from build123d import *

# Parameters (mm, degrees)
SKETCH1_R           = 50
BOSS_EXTRUDE1_DEPTH = 80
BOSS_EXTRUDE2_START = 4
SKETCH1_3_R         = 56
SKETCH1_3_R_2       = 50
BOSS_EXTRUDE2_DEPTH = 4
SKETCH5_W           = 51
SKETCH5_H           = 28
BOSS_EXTRUDE4_DEPTH = 38
SKETCH6_W           = 47
SKETCH6_H           = 28
CUT_EXTRUDE2_DEPTH  = 36
SKETCH8_R           = 7.5
CUT_EXTRUDE3_DEPTH  = 51


with BuildPart() as part:
    # Sketch1 → Boss-Extrude1 (new body)
    with BuildSketch(Plane(origin=(0, 0, 0), x_dir=(1, 0, 0), z_dir=(0, 1, 0))):
        with Locations(Location((0, 0, 0), (0, 0, 270))):
            Circle(SKETCH1_R)
    extrude(amount=-BOSS_EXTRUDE1_DEPTH)

    # Sketch1_3 → Boss-Extrude2 (add)
    # profile 1 of 2: a face of its own
    with BuildSketch(Plane(origin=(0, 0, 0), x_dir=(1, 0, 0), z_dir=(0, 1, 0)).offset(BOSS_EXTRUDE2_START)):
        with Locations(Location((0, 0, 0), (0, 0, 270))):
            Circle(SKETCH1_3_R)
        with Locations(Location((0, 0, 0), (0, 0, 270))):
            Circle(SKETCH1_3_R_2, mode=Mode.SUBTRACT)
    # profile 2 of 2: a face of its own
    with BuildSketch(Plane(origin=(0, 0, 0), x_dir=(1, 0, 0), z_dir=(0, 1, 0)).offset(BOSS_EXTRUDE2_START)):
        with Locations(Location((0, 0, 0), (0, 0, 270))):
            Circle(SKETCH1_3_R_2)
    extrude(amount=-BOSS_EXTRUDE2_DEPTH)

    # Sketch5 → Boss-Extrude4 (add)
    with BuildSketch(Plane(origin=(0, 4, 0), x_dir=(1, 0, 0), z_dir=(0, 1, 0))):
        Rectangle(SKETCH5_W, SKETCH5_H)
    extrude(amount=BOSS_EXTRUDE4_DEPTH)

    # Sketch6 → Cut-Extrude2 (cut)
    with BuildSketch(Plane(origin=(0, 42, 0), x_dir=(1, 0, 0), z_dir=(0, 1, 0))):
        Rectangle(SKETCH6_W, SKETCH6_H)
    extrude(amount=-CUT_EXTRUDE2_DEPTH, mode=Mode.SUBTRACT)

    # Sketch8 → Cut-Extrude3 (cut)
    with BuildSketch(Plane(origin=(25.5, 0, 0), x_dir=(0, 0, -1), z_dir=(1, 0, 0))):
        with Locations((0, 42)):
            Circle(SKETCH8_R)
    extrude(amount=-CUT_EXTRUDE3_DEPTH, mode=Mode.SUBTRACT)


solid = part.part
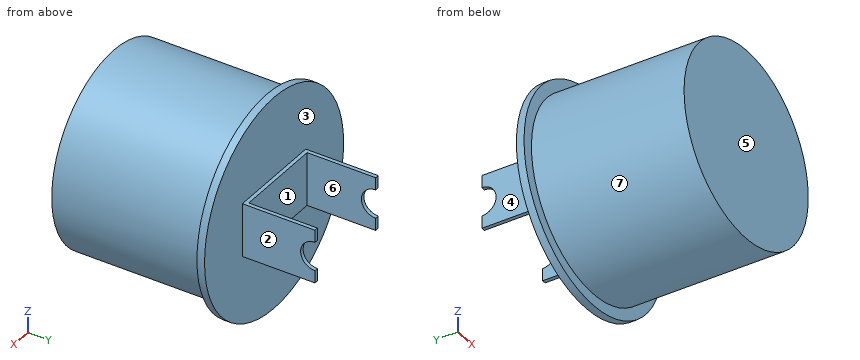
Part model, mm, in its own coordinate system. Face numbers are marked on the shaded views. A direction names the side the tool comes from. Give positions to 0.01 mm unless a question says otherwise; leave off trailing zeros. Order: outer loops, then holes, each group sorted by start corner. A loop starts at its lowest first (then second) coordinate and runs counter-clockwise, first axis right, second up. Notation, with made-up numbers: (-31.75, 36) - (4.25, 36) arc R28 cw to (4.25, 71) - close; hole circle Ø6 at (-25.5, 19.25). An arc over 180 degrees is marked (long way). One line per question, with ' | ' between items.
1. Band-saw the part on C-C on y = -57. List the corners of the cut face in (x, z).
Filled in:
outline: circle Ø100 at (0, 0)
2. Band-saw the part on D-D on z = 34. List the corners of the cut face in (x, y).
Filled in:
outline: (-44.5, 0) - (-36.66, 0) - (-36.66, -80) - (36.66, -80) - (36.66, 0) - (44.5, 0) - (44.5, 4) - (-44.5, 4) - close
3. Pull direction X, two halves, no side cores. Call the marked faces 1, 2 and 3: +X half, -X half, draft (parallel to the pull), parting line (faces both ways), or undercut.
Filled in:
face 1: undercut | face 2: +X half | face 3: draft
4. Drop flat-ended pins along their axis: P1, Ø8.5, axis at y = 28.5, z = 1, coming from the -X side; P2, Ø14, axis at x = 7.5, z = 0, coming from the +Y side; P3, Ø10, axis at y = -62.5, z = -30.5, coming from the -X side. Give the stop position or say it passes through.
Filled in:
P1: x = -25.5 | P2: y = 6 | P3: x = -43.01
5. Band-saw the part on A-A on x = 0. List the corners of the cut face in (y, z), then the cut area to 3 significant figures.
Filled in:
outline: (-80, -50) - (0, -50) - (0, -56) - (4, -56) - (4, -14) - (6, -14) - (6, 14) - (4, 14) - (4, 56) - (0, 56) - (0, 50) - (-80, 50) - close | area: 8,500 mm²
6. Drill centre lines: probe 1 along Y at (x, z) = (45.5, 30.5); probe 2 along Y at (x, z) = (7, -4); probe 3 along X at (y, z) = (-72.5, 1.5). Where is each one in solid material? Low to high.
Filled in:
probe 1: 0 to 4 | probe 2: -80 to 6 | probe 3: -49.98 to 49.98
7. Band-saw the part on B-B on z = 0. List the corners of the cut face in (x, y).
Filled in:
outline: (-56, 0) - (-50, 0) - (-50, -80) - (50, -80) - (50, 0) - (56, 0) - (56, 4) - (25.5, 4) - (25.5, 34.5) - (23.5, 34.5) - (23.5, 6) - (-23.5, 6) - (-23.5, 34.5) - (-25.5, 34.5) - (-25.5, 4) - (-56, 4) - close
8. Which spindle directions (+Z, -Z, +X, -X, +Y, -Y) get a long thin tool onto all of the face, cutting with end or side? Do the marked faces 4, 5, 6 and 7. Say none if no direction does.
Filled in:
face 4: +Z, -Z, -X, +Y | face 5: +Z, -Z, +X, -X, -Y | face 6: +Z, -Z, +Y | face 7: -Y
